```python
from build123d import *

# Parameters (mm, degrees)
F1_DEPTH = 3.175
F3_DEPTH = 3.175
F4_R     = 9.5504
F5_DEPTH = 3.2258
F6_R     = 3.175
F7_DEPTH = 6.351


with BuildPart() as f1:
    # F0 (on Top) → F1 (new body)
    with BuildSketch(Plane.XY):
        with BuildLine():
            ThreePointArc((2.117, -12.522313), (9.699894, -8.197686), (12.7, 0))
            ThreePointArc((12.7, 0), (9.699894, 8.197686), (2.117, 12.522313))
            ThreePointArc((2.117, 12.522313), (-12.7, 0), (2.117, -12.522313))
        make_face()
        with BuildLine():
            ThreePointArc((2.117, 12.522313), (9.699894, 8.197686), (12.7, 0))
            ThreePointArc((12.7, 0), (9.699894, -8.197686), (2.117, -12.522313))
            Line((2.117, -12.522313), (39.047233, -6.278953))
            ThreePointArc((39.047233, -6.278953), (31.75, 0), (39.047233, 6.278953))
            Line((39.047233, 6.278953), (2.117, 12.522313))
        make_face()
        with BuildLine():
            ThreePointArc((44.45, 0), (42.913389, 4.141713), (39.047233, 6.278953))
            ThreePointArc((39.047233, 6.278953), (31.75, 0), (39.047233, -6.278953))
            ThreePointArc((39.047233, -6.278953), (42.913389, -4.141713), (44.45, 0))
        make_face()
    extrude(amount=F1_DEPTH)

    # F2 (on face) → F3 (join)
    with BuildSketch(Plane.XY.offset(3.175)):
        with BuildLine():
            ThreePointArc((39.047233, 6.278953), (31.75, 0), (39.047233, -6.278953))
            ThreePointArc((39.047233, -6.278953), (42.913389, -4.141713), (44.45, 0))
            ThreePointArc((44.45, 0), (42.913389, 4.141713), (39.047233, 6.278953))
        make_face()
        with BuildLine():
            ThreePointArc((12.7, 0), (9.699894, 8.197686), (2.117, 12.522313))
            ThreePointArc((2.117, 12.522313), (-12.7, 0), (2.117, -12.522313))
            ThreePointArc((2.117, -12.522313), (9.699894, -8.197686), (12.7, 0))
        make_face()
    extrude(amount=F3_DEPTH)

    # F4 (on face) → F5 (cut)
    with BuildSketch(Plane.XY.offset(6.35)):
        Circle(F4_R)
    extrude(amount=-F5_DEPTH, mode=Mode.SUBTRACT)

    # F6 (on face) → F7 (cut, through all)
    with BuildSketch(Plane.XY.offset(6.35)):
        with Locations((38.1, 0)):
            Circle(F6_R)
    extrude(amount=-F7_DEPTH, mode=Mode.SUBTRACT)


solid = f1.part
```
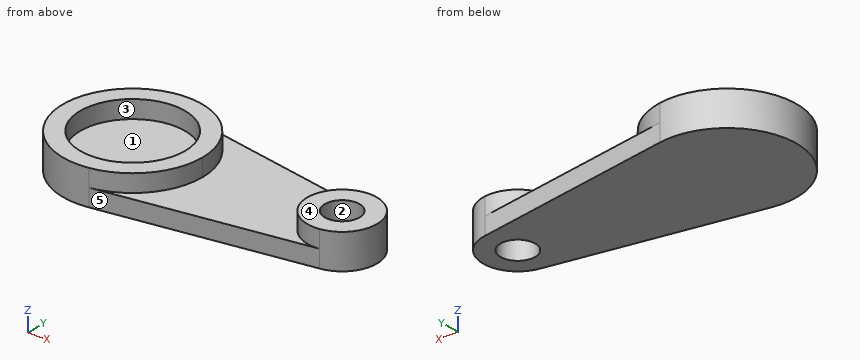
Here's how the part is built. I have some questions about the finished solid (model axes, mm). Face numbers are marked on the shaded views. A direction names the side the tool comes from. Round coordinates to 2 decimals unless told otherwise and drop trailing zeros. Loops run counter-clockwise (first coordinate to the right, second up) from the corner with the lowest first, then second, coordinate; pieces in that order, holes last. Notation, with made-up numbers: (-19, 18.25) -> (-15, 18.25) arc R13 cw to (-15, 23.25) -> close; hole circle Ø8 at (-21, 7.5). An arc over 180 degrees is marked (long way). Answer as CSV lines item,"result". Start each with the question number.
1. Imagine slicing it at C-C on x = 38.1. Write out the boundary of the cut face in (y, z) (3 decimals).
2. For the marked faces 1 and 2, which set-ups out of +Z, -Z, +X, -X, +Y, -Y let a thin tool reach every point of the face, with its end or its side?
3. I need wall thicknesses on probe 1 along Y at (x, z) = (0, 5.2); probe 2 along Y at (x, z) = (38.1, 4.5) (3 decimals); probe 3 along X at (y, z) = (2.25, 3.25). Which ranges of each line are inside material? Lowest first, please. Write a range as from..to.
4. If we mould it in two halves opening along X, with no side actions, what happens to the marked faces 3, 4 and 5? For each: pulls with the +X half, pulls with the -X half, needs draft (parallel to the pull), parting line crosses it, or undercut.
5. Imagine slicing it at B-B on x = 0. Write out the boundary of the cut face in (y, z), plus the area to 3 significant figures.
6. Imagine slicing it at A-A on z = 5. Write out the boundary of the cut face in (x, y) (3 decimals), plus the area to 3 significant figures.
7. Imagine slicing it at D-D on z = 1.5. Write out the boundary of the cut face in (x, y) (3 decimals).
8. I'm going to push flat-ended pins straight in: P1, Ø7.5, axis at x = 38.1, y = 0, coming from the -Z side; P2, Ø1, axis at y = -3, z = 0.5, coming from the +X side; P3, Ø2, axis at x = 7, z = 3.5, coming from the +Y side; P4, Ø3, axis at x = 2, z = 3.5, coming from the +Y side. Where does each tip first touch, or does it pass through?
Solution:
1,outline,"(-6.439, 0) -> (-3.175, 0) -> (-3.175, 6.35) -> (-6.35, 6.35) -> (-6.35, 3.175) -> (-6.439, 3.175) -> close; (3.175, 0) -> (6.439, 0) -> (6.439, 3.175) -> (6.35, 3.175) -> (6.35, 6.35) -> (3.175, 6.35) -> close"
2,face 1,"+Z"
2,face 2,"+Z, -Z"
3,probe 1,"-12.7..-9.55, 9.55..12.7"
3,probe 2,"-6.35..-3.175, 3.175..6.35"
3,probe 3,"-12.5..-9.28, 9.28..12.5, 32.16..35.86, 40.34..44.04"
4,face 3,"undercut"
4,face 4,"needs draft"
4,face 5,"pulls with the +X half"
5,outline,"(-12.7, 0) -> (12.7, 0) -> (12.7, 6.35) -> (9.55, 6.35) -> (9.55, 3.12) -> (-9.55, 3.12) -> (-9.55, 6.35) -> (-12.7, 6.35) -> close"
5,area,"99.7 mm²"
6,outline,"(2.117, -12.522) arc R12.7 ccw to (2.117, 12.522) arc R12.7 ccw (long way) to start; circle Ø12.7 at (38.1, 0); hole circle Ø19.101 at (0, 0); hole circle Ø6.35 at (38.1, 0)"
6,area,"315 mm²"
7,outline,"(2.117, -12.522) -> (39.047, -6.279) arc R6.35 ccw to (39.047, 6.279) -> (2.117, 12.522) arc R12.7 ccw (long way) to start; hole circle Ø6.35 at (38.1, 0)"
8,P1,"z = 0"
8,P2,"x = 43.94"
8,P3,"y = 11.86"
8,P4,"y = 12.69"
